Geometry check sheet. Reference: drawing and pictorial views, mm from the part's lowest x, y, z. Coordinates: 2 decimals unless noted, no trailing zeros. Loops run counter-clockwise (first coordinate to the right, second up) from the corner with the lowest first, then second, coordinate; pieces in that order, holes last.
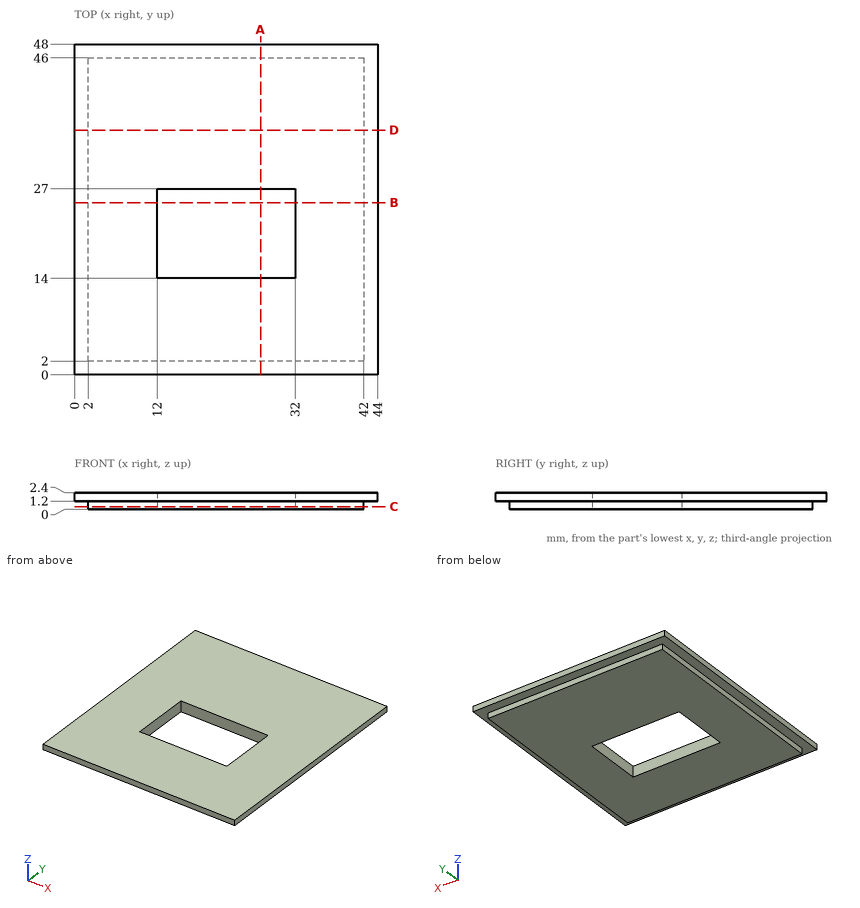
1) Section check A-A on x = 27. Record the cut outline in (y, z), and give its area (3 significant figures).
Data:
outline: (0, 1.2) - (2, 1.2) - (2, 0) - (14, 0) - (14, 2.4) - (0, 2.4) - close; (27, 0) - (46, 0) - (46, 1.2) - (48, 1.2) - (48, 2.4) - (27, 2.4) - close
area: 79.2 mm2
2) Material ranges on probe 1 along Y at (x, z) = (24, 2.05); probe 2 along X at (y, z) = (18, 0.75); probe 3 along Y at (x, z) = (19.5, 0.55), recorded low to high.
Data:
probe 1: y = 0 to 14, 27 to 48
probe 2: x = 2 to 12, 32 to 42
probe 3: y = 2 to 14, 27 to 46
3) Section check C-C on z = 0.4. Record the cut outline in (x, y), and give its area (3 significant figures).
Data:
outline: (2, 2) - (42, 2) - (42, 46) - (2, 46) - close; hole (12, 14) - (32, 14) - (32, 27) - (12, 27) - close
area: 1,500 mm2
4) Section check B-B on y = 25. Record the cut outline in (x, z).
Data:
outline: (0, 1.2) - (2, 1.2) - (2, 0) - (12, 0) - (12, 2.4) - (0, 2.4) - close; (32, 0) - (42, 0) - (42, 1.2) - (44, 1.2) - (44, 2.4) - (32, 2.4) - close
5) Depth check by flat-ended pin: pin 1 (1 mm diameter, centred on y = 21.5, z = 0.5, fed in from +X); pin 2 (1.3 mm diameter, centred on y = 30.5, z = 0.5, fed in from -X); pin 3 (1.3 mm diameter, centred on x = 29.5, z = 0.5, fed in from +Y); pin 4 (10 mm diameter, centred on x = 32, y = 6.5, fed in from -Z). Enter the tip coordinate at first touch or a pass-through.
Data:
pin 1: stops at x = 42
pin 2: stops at x = 2
pin 3: stops at y = 46
pin 4: stops at z = 0
6) Section check D-D on y = 35.5. Record the cut outline in (x, z), and give its area (3 significant figures).
Data:
outline: (0, 1.2) - (2, 1.2) - (2, 0) - (42, 0) - (42, 1.2) - (44, 1.2) - (44, 2.4) - (0, 2.4) - close
area: 101 mm2
